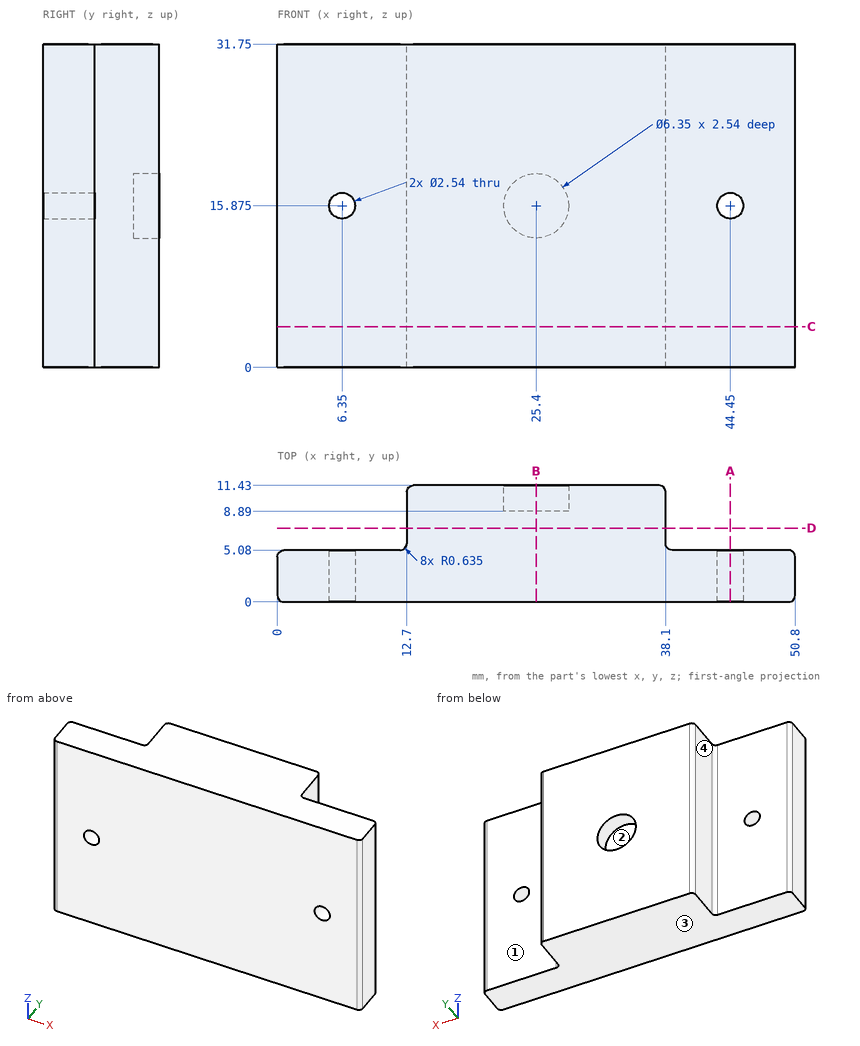
Geometry: see drawing. Coordinates: mm, zero at the bounding-box minimum. A direction names the side the tool comes from. Coordinates: 2 decimals unless noted, no trailing zeros. Loops run counter-clockwise (first coordinate to the right, second up) from the corner with the lowest first, then second, coordinate; pieces in that order, holes last. Notation, with made-up numbers: M 76,12 L 135,12 A17 ccw 135,37 Z; hole C 3.5,32 d9. An arc over 180 degrees is marked long. Put each result on its own line as item: value. Start each with the question number.
1) Cut plane B-B on x = 25.4. Return the cut outline in (y, z).
2) Cut plane A-A on x = 44.45. Return the cut outline in (y, z) (3 decimals), then the cut area to 3 significant figures.
3) Reachability of the marked faces 1, 2, 3 and 4 from +Z, -Z, +X, -X, +Y, -Y: full face, straight path, thin tool, end or side. Return the list, or none.
4) Ray query, L1, parallel to Z at x = 6.35, y = 1.35 (3 decimals); L2, parallel to Y at x = 41, z = 8; L3, parallel to X at y = 9.5, z = 29.5. Return the intervals inside material, ascending. Write a range as from..to.
5) Cut plane D-D on y = 7.25. Return the cut outline in (x, z).
6) Contact query for flat-ended pins moving along their axis: pin 1 Ø1.5 at (y, z) = (8.5, 19) entering from -X; pin 2 Ø1.9 at (x, z) = (24.5, 14.5) entering from +Y; pin 3 Ø4 at (y, z) = (8, 11.5) entering from +X. Output: stop coordinate, or through.
7) Cut plane C-C on z = 4. Return the cut outline in (x, y) (3 decimals), then the cut area to 3 significant figures.
The answers:
1. outline: M 0,0 L 11.43,0 L 11.43,12.7 L 8.89,12.7 L 8.89,19.05 L 11.43,19.05 L 11.43,31.75 L 0,31.75 Z
2. outline: M 0,0 L 5.08,0 L 5.08,14.605 L 0,14.605 Z; M 0,17.145 L 5.08,17.145 L 5.08,31.75 L 0,31.75 Z
2. area: 148 mm²
3. face 1: +Z, -Z, +X, +Y
3. face 2: +Y
3. face 3: -Z, +X, -X, +Y, -Y
3. face 4: +Z, -Z, -X, +Y
4. L1: z = 0..14.605, 17.145..31.75
4. L2: y = 0..5.08
4. L3: x = 12.7..38.1
5. outline: M 12.7,0 L 38.1,0 L 38.1,31.75 L 12.7,31.75 Z
6. pin 1: stops at x = 12.7
6. pin 2: stops at y = 8.89
6. pin 3: stops at x = 38.1
7. outline: M 0,0.635 A0.635 ccw 0.635,0 L 50.165,0 A0.635 ccw 50.8,0.635 L 50.8,4.445 A0.635 ccw 50.165,5.08 L 38.735,5.08 A0.635 cw 38.1,5.715 L 38.1,10.795 A0.635 ccw 37.465,11.43 L 13.335,11.43 A0.635 ccw 12.7,10.795 L 12.7,5.715 A0.635 cw 12.065,5.08 L 0.635,5.08 A0.635 ccw 0,4.445 Z
7. area: 419 mm²
